```python
from build123d import *

# Parameters (mm, degrees)
SKETCH1_R           = 15
BOSS_EXTRUDE1_DEPTH = 40
SKETCH2_W           = 10
SKETCH2_H           = 30
BOSS_EXTRUDE2_DEPTH = 40
SKETCH3_R           = 7.5
CUT_EXTRUDE1_DEPTH  = 40
FILLET2_R           = 10


with BuildPart() as part:
    # Sketch1 → Boss-Extrude1 (new body)
    with BuildSketch(Plane(origin=(0, 0, 0), x_dir=(1, 0, 0), z_dir=(0, 1, 0))):
        with Locations(Location((0, 0, 0), (0, 0, 270))):
            Circle(SKETCH1_R)
    extrude(amount=BOSS_EXTRUDE1_DEPTH)

    # Sketch2 → Boss-Extrude2 (add)
    with BuildSketch(Plane.XZ):
        Rectangle(SKETCH2_W, SKETCH2_H)
    extrude(amount=BOSS_EXTRUDE2_DEPTH)

    # Sketch3 → Cut-Extrude1 (cut)
    with BuildSketch(Plane.ZY.offset(5)):
        with Locations((0, -30)):
            Circle(SKETCH3_R)
    extrude(amount=-CUT_EXTRUDE1_DEPTH, mode=Mode.SUBTRACT)

    # Fillet2
    fillet2_edges = [part.edges().sort_by_distance(p)[0] for p in [
        (0, -40, 15),
        (0, -40, -15),
    ]]
    fillet(fillet2_edges, radius=FILLET2_R)


solid = part.part
```
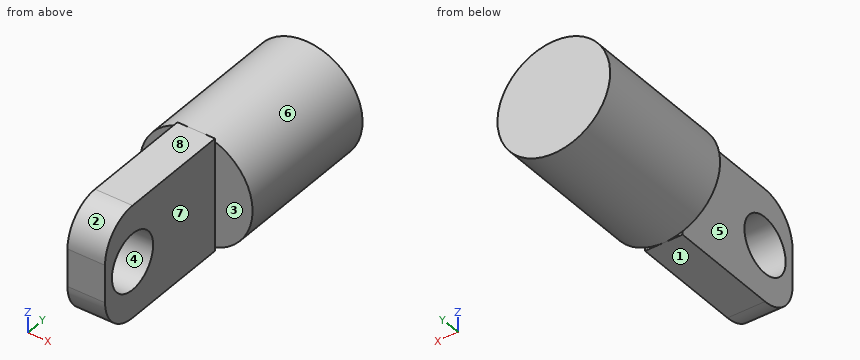
Verification items for the finished model (mm, model axes). Face numbers are marked on the shaded views. A direction names the side the tool comes from. Coordinates: 2 decimals unless noted, no trailing zeros. Order: outer loops, then holes, each group sorted by start corner. A loop starts at its lowest first (then second) coordinate and runs counter-clockwise, first axis right, second up. Notation, with made-up numbers: (59, 48) -> (118, 48) arc R13 cw to (118, 70) -> close; hole circle Ø3 at (35, -6). An arc over 180 degrees is marked (long way). Answer as CSV lines item,"result". Start each with the question number.
1) Cross-section at A-A, the plane z = 0. Record the boundary of the cut face in (x, y).
2) Cross-section at B-B, the plane y = -33.5. Record the boundary of the cut face in (x, z).
3) Gauge pin test, flat ends, axial feed: pin 1 Ø11 at (x, z) = (11, -2) entering from -Y; pin 2 Ø8 at (y, z) = (6, 8.5) entering from -X; pin 3 Ø9 at (y, z) = (-29, -0.5) entering from +X; pin 4 Ø6 at (y, z) = (-17, -2.5) entering from +X. Record the tip position at first contact, or that the pin passes through.
4) Set-up check for the marked faces 5, 6, 7 and 8: record each of +Z, -Z, +X, -X, +Y, -Y from which the full face is reachable in a straight line by a thin tool's end or side.
5) Material ranges on L1, parallel to Y at x = -1.75, z = 0; L2, parallel to X at y = -12, z = 9; L3, parallel to Y at x = -12, z = 6.5, recorded low to high. Write a range as [from, to].
6) Release check for a two-part mould opening along Z. For the marked faces 1, 2, 3 and 4 record: released by +Z, released by -Z, zero draft, split by the parting line, or undercut.
7) Cross-section at D-D, the plane z = -11. Record the boundary of the cut face in (x, y), then the cut area to 3 significant figures.
Conclusion:
1,outline,"(-15, 0) -> (-5, 0) -> (-5, -22.5) -> (5, -22.5) -> (5, 0) -> (15, 0) -> (15, 40) -> (-15, 40) -> close; (-5, -40) -> (5, -40) -> (5, -37.5) -> (-5, -37.5) -> close"
2,outline,"(-5, -14.37) -> (5, -14.37) -> (5, -6.63) -> (-5, -6.63) -> close; (-5, 6.63) -> (5, 6.63) -> (5, 14.37) -> (-5, 14.37) -> close"
3,pin 1,"stops at y = 0"
3,pin 2,"stops at x = -14.31"
3,pin 3,"passes through"
3,pin 4,"stops at x = 5"
4,face 5,"+Z, -Z, -X, -Y"
4,face 6,"+Y"
4,face 7,"+Z, -Z, +X, -Y"
4,face 8,"+Z, +X, -X, +Y, -Y"
5,L1,"y = [-40, -37.5], [-22.5, 40]"
5,L2,"x = [-5, 5]"
5,L3,"y = [0, 40]"
6,face 1,"released by -Z"
6,face 2,"released by +Z"
6,face 3,"zero draft"
6,face 4,"undercut"
7,outline,"(-10.2, 0) -> (-5, 0) -> (-5, -38) -> (5, -38) -> (5, 0) -> (10.2, 0) -> (10.2, 40) -> (-10.2, 40) -> close"
7,area,"1,200 mm²"
